The model under review builds one solid part; all positions refer to its coordinate system, in mm. Face numbers are marked on the shaded views. A direction names the side the tool comes from. Give positions to 0.01 mm unless a question says otherwise; leave off trailing zeros. Loops run counter-clockwise (first coordinate to the right, second up) from the corner with the lowest first, then second, coordinate; pieces in that order, holes last. Notation, with made-up numbers: M -19.75,-30 L 35.25,-30 A23 cw 35.25,-11 Z; hole C -24,47 d6. An arc over 180 degrees is marked long. Write item = value, one per line. Start each with the question number.
1. We need section A-A on x = 4.25. Give the boundary of the cut face in (y, z) (3 decimals), then the cut area to 3 significant figures.
2. We need section C-C on z = 6. Count the separate pieces of the cut face and the enclosed holes in it, then the cut area to 3 significant figures.
3. Wall thickness on line 1 along Y through (x, z) = (4.25, -5.5); line 2 along Y through (x, z) = (7, -2.5); line 3 along Z through (x, y) = (5.75, 4.5): over which ranges is each line inside the solid? List them lowest first. Write a range as from..to.
4. Draft analysis for pull direction Y (two halves, no side actions). For the marked faces 1, 2 and 3, state which applies: pulls with the +Y half, pulls with the -Y half, needs draft (parallel to the pull), parting line crosses it, or undercut.
5. For pin 1 (3 mm diameter, centred on x = 19, z = 0, fed in from -Y); pin 2 (10 mm diameter, centred on x = 8.5, y = 18, fed in from -Z); pin 3 (5 mm diameter, centred on y = 12, z = -9.5, fed in from +X), all flat-tipped, find the tip position at first contact; note any pin that passes through.
6. We need section D-D on x = 14. Give the boundary of the cut face in (y, z), then the cut area to 3 significant figures.
7. For the marked faces 4 and 5, list the 3-axis set-ups (+Z, -Z, +X, -X, +Y, -Y) from which the entire face can be reached by the end or side of a thin tool; tool diameter is ignored.
8. We need section B-B on x = 7.75. Give the boundary of the cut face in (y, z) (3 decimals), then the cut area to 3 significant figures.
from build123d import *

# Parameters (mm, degrees)
CUT_EXTRUDE_2_DEPTH = 6
CUT_EXTRUDE_3_DEPTH = 26
SKETCH_3_R          = 6.5
CUT_EXTRUDE_4_DEPTH = 26
CHAMFER_1_SIZE      = 1
CHAMFER_3_SIZE      = 1


with BuildPart() as part:
    # Эскиз1 → Повернуть1 (revolve)
    with BuildSketch(Plane.XY):
        Polygon((0, 0), (0, 24), (1, 25), (9, 25), (10, 24), (10, 10), (24, 10), (25, 9), (25, 0), align=None)
    revolve(axis=Axis((0, 0, 0), (1, 0, 0)))

    # Эскиз4 → Вырез-Вытянуть2 (cut)
    with BuildSketch(Plane.ZY):
        with BuildLine():
            ThreePointArc((7.875, 19.467521029), (0, 21), (-7.875, 19.467521029))
            ThreePointArc((-7.875, 19.467521029), (-10.635124054, 12.957396974), (-4.125, 10.19727292))
            ThreePointArc((-4.125, 10.19727292), (0, 11), (4.125, 10.19727292))
            ThreePointArc((4.125, 10.19727292), (10.635124054, 12.957396974), (7.875, 19.467521029))
        make_face()
        with BuildLine():
            ThreePointArc((-10.19727292, 4.125), (-11, 0), (-10.19727292, -4.125))
            ThreePointArc((-10.19727292, -4.125), (-12.957396974, -10.635124054), (-19.467521029, -7.875))
            ThreePointArc((-19.467521029, -7.875), (-21, 0), (-19.467521029, 7.875))
            ThreePointArc((-19.467521029, 7.875), (-12.957396974, 10.635124054), (-10.19727292, 4.125))
        make_face()
        with BuildLine():
            ThreePointArc((-4.125, -10.19727292), (0, -11), (4.125, -10.19727292))
            ThreePointArc((4.125, -10.19727292), (10.635124054, -12.957396974), (7.875, -19.467521029))
            ThreePointArc((7.875, -19.467521029), (0, -21), (-7.875, -19.467521029))
            ThreePointArc((-7.875, -19.467521029), (-10.635124054, -12.957396974), (-4.125, -10.19727292))
        make_face()
    extrude(amount=-CUT_EXTRUDE_2_DEPTH, mode=Mode.SUBTRACT)

    # Эскиз5 → Вырез-Вытянуть3 (cut, through all)
    with BuildSketch(Plane.ZY):
        with BuildLine():
            ThreePointArc((7.125, 17.613471407), (0, 19), (-7.125, 17.613471407))
            ThreePointArc((-7.125, 17.613471407), (-8.781074433, 13.707396974), (-4.875, 12.051322542))
            ThreePointArc((-4.875, 12.051322542), (0, 13), (4.875, 12.051322542))
            ThreePointArc((4.875, 12.051322542), (8.781074433, 13.707396974), (7.125, 17.613471407))
        make_face()
        with BuildLine():
            ThreePointArc((-12.051322542, 4.875), (-13, 0), (-12.051322542, -4.875))
            ThreePointArc((-12.051322542, -4.875), (-13.707396974, -8.781074433), (-17.613471407, -7.125))
            ThreePointArc((-17.613471407, -7.125), (-19, 0), (-17.613471407, 7.125))
            ThreePointArc((-17.613471407, 7.125), (-13.707396974, 8.781074433), (-12.051322542, 4.875))
        make_face()
        with BuildLine():
            ThreePointArc((-4.875, -12.051322542), (0, -13), (4.875, -12.051322542))
            ThreePointArc((4.875, -12.051322542), (8.781074433, -13.707396974), (7.125, -17.613471407))
            ThreePointArc((7.125, -17.613471407), (0, -19), (-7.125, -17.613471407))
            ThreePointArc((-7.125, -17.613471407), (-8.781074433, -13.707396974), (-4.875, -12.051322542))
        make_face()
    extrude(amount=-CUT_EXTRUDE_3_DEPTH, mode=Mode.SUBTRACT)

    # Эскиз3 → Вырез-Вытянуть4 (cut, through all)
    with BuildSketch(Plane(origin=(25, 0, 0), x_dir=(0, 0, -1), z_dir=(1, 0, 0))):
        with Locations((-0.5, 0)):
            Circle(SKETCH_3_R)
    extrude(amount=-CUT_EXTRUDE_4_DEPTH, mode=Mode.SUBTRACT)

    # Фаска1
    chamfer_1_edges = [part.edges().sort_by_distance(p)[0] for p in [
        (25, 0, 7),
    ]]
    chamfer(chamfer_1_edges, length=CHAMFER_1_SIZE)

    # Фаска3
    chamfer_3_edges = [part.edges().sort_by_distance(p)[0] for p in [
        (0, 0, 7),
    ]]
    chamfer(chamfer_3_edges, length=CHAMFER_3_SIZE)


solid = part.part
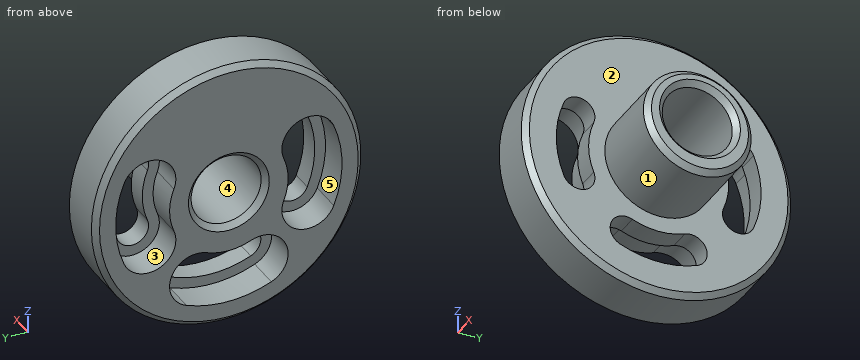
Final values:
q1.outline = C 0,0 d50; hole M -19.468,-7.875 A5 ccw -10.197,-4.125 A11 cw -10.197,4.125 A5 ccw -19.468,7.875 A21 ccw Z; hole M -7.875,-19.468 A21 ccw 7.875,-19.468 A5 ccw 4.125,-10.197 A11 cw -4.125,-10.197 A5 ccw Z; hole C 0,0.5 d13; hole M 10.197,-4.125 A5 ccw 19.468,-7.875 A21 ccw 19.468,7.875 A5 ccw 10.197,4.125 A11 cw Z
q1.area = 1,230 mm²
q2.separate_pieces = 4
q2.enclosed_holes = 0
q2.area = 372 mm²
q3.line_1 = -24.39..-20.27, -9.86..-2.5, 2.5..9.86, 20.27..24.39
q3.line_2 = -24.87..-18.83, -12.76..-5.77, 5.77..12.76, 18.83..24.87
q3.line_3 = -24.59..-20.51, -10.06..-4.19, 5.19..24.59
q4.face_1 = parting line crosses it
q4.face_2 = needs draft
q4.face_3 = undercut
q5.pin_1 = -10
q5.pin_2 = -21.35
q5.pin_3 = 10
q6.outline = C 0,0 d20; hole C 0,0.5 d13
q6.area = 181 mm²
q7.face_4 = +X, -X
q7.face_5 = -X
q8.outline = C 0,0 d50; hole M -17.613,-7.125 A3 ccw -12.051,-4.875 A13 cw -12.051,4.875 A3 ccw -17.613,7.125 A19 ccw Z; hole M -7.125,-17.613 A19 ccw 7.125,-17.613 A3 ccw 4.875,-12.051 A13 cw -4.875,-12.051 A3 ccw Z; hole C 0,0.5 d13; hole M 12.051,-4.875 A3 ccw 17.613,-7.125 A19 ccw 17.613,7.125 A3 ccw 12.051,4.875 A13 cw Z
q8.area = 1,520 mm²
